from build123d import *

# Parameters (mm, degrees)
SKETCH_1_R      = 11
SKETCH_1_R_2    = 1.5
SKETCH_1_R_3    = 3
EXTRUDE_1_DEPTH = 4


with BuildPart() as part:
    # 草图1 → 凸台-拉伸1 (new body)
    with BuildSketch(Plane.XY):
        with BuildLine():
            Line((-15.909902577, 23.909902577), (15.909902577, 23.909902577))
            ThreePointArc((15.909902577, 23.909902577), (21.566756826, 21.566756826), (23.909902577, 15.909902577))
            Line((23.909902577, 15.909902577), (23.909902577, -15.909902577))
            ThreePointArc((23.909902577, -15.909902577), (21.566756826, -21.566756826), (15.909902577, -23.909902577))
            Line((15.909902577, -23.909902577), (-15.909902577, -23.909902577))
            ThreePointArc((-15.909902577, -23.909902577), (-21.566756826, -21.566756826), (-23.909902577, -15.909902577))
            Line((-23.909902577, -15.909902577), (-23.909902577, 15.909902577))
            ThreePointArc((-23.909902577, 15.909902577), (-21.566756826, 21.566756826), (-15.909902577, 23.909902577))
        make_face()
        Circle(SKETCH_1_R, mode=Mode.SUBTRACT)
        with Locations((0, 14)):
            Circle(SKETCH_1_R_2, mode=Mode.SUBTRACT)
        with Locations((14, 0)):
            Circle(SKETCH_1_R_2, mode=Mode.SUBTRACT)
        with Locations((0, -14)):
            Circle(SKETCH_1_R_2, mode=Mode.SUBTRACT)
        with Locations((-14, 0)):
            Circle(SKETCH_1_R_2, mode=Mode.SUBTRACT)
        with Locations((15.909902577, 15.909902577)):
            Circle(SKETCH_1_R_3, mode=Mode.SUBTRACT)
        with Locations((15.909902577, -15.909902577)):
            Circle(SKETCH_1_R_3, mode=Mode.SUBTRACT)
        with Locations((-15.909902577, -15.909902577)):
            Circle(SKETCH_1_R_3, mode=Mode.SUBTRACT)
        with Locations((-15.909902577, 15.909902577)):
            Circle(SKETCH_1_R_3, mode=Mode.SUBTRACT)
    extrude(amount=EXTRUDE_1_DEPTH)


solid = part.part
The listing builds one solid part. Answer for the finished solid, in the listing's coordinates (mm). Coordinates: 2 decimals unless noted, no trailing zeros. Write each loop counter-clockwise with the first axis right and the second up, starting at its lowest first coordinate (ties: lowest second). Pieces come first, ordered by that corner, then holes. Notation, with made-up numbers: (19.25, 42.25) -> (47.25, 42.25) arc R17 ccw to (47.25, 62.25) -> close; hole circle Ø5 at (32.5, -17). An arc over 180 degrees is marked (long way). One line per question, with ' | ' between items.
1. Section D-D (y = 7.5) is taken. Determine the outline of the cut face in (x, z), and give its area (3 significant figures).
Verdict:
outline: (-23.91, 0) -> (-8.05, 0) -> (-8.05, 4) -> (-23.91, 4) -> close; (8.05, 0) -> (23.91, 0) -> (23.91, 4) -> (8.05, 4) -> close | area: 127 mm^2
2. Section B-B (z = 2.3) is taken. State how many separate pieces and enclosed holes the cut face has, and give its area (3 significant figures).
Verdict:
separate pieces: 1 | enclosed holes: 9 | area: 1,710 mm^2
3. Given pin 1 Ø2 at (y, z) = (18.5, 1.5) entering from -X; pin 2 Ø1 at (x, z) = (-18, 2.5) entering from +Y, each flat-ended and moving along its own axis, determine where each tip first touches the part or whether it passes through.
Verdict:
pin 1: stops at x = -23.75 | pin 2: stops at y = 23.75
4. Straight lines are drawn through the part: line 1 (X direction, y = -16, z = 1.15); line 2 (Y direction, x = 0, z = 3); line 3 (Y direction, x = -14, z = 2.2). For each, find the intervals that lie inside material, in ascending order.
Verdict:
line 1: x = -23.91 to -18.91, -12.91 to 12.91, 18.91 to 23.91 | line 2: y = -23.91 to -15.5, -12.5 to -11, 11 to 12.5, 15.5 to 23.91 | line 3: y = -23.91 to -18.22, -13.6 to -1.5, 1.5 to 13.6, 18.22 to 23.91
5. For a pull along Y with two mould halves and no side action, classify faces 1 (the flat face through (0, 23.91, 2)), 2 (the cylindrical face through (-0.325, 12.536, 1.972)), 3 (the cylindrical face through (21.63, -21.5, 1.97)), 4 (the cylindrical face through (15.26, -18.84, 1.97)) as released by +Y, released by -Y, zero draft, split by the parting line, or undercut.
Verdict:
face 1: released by +Y | face 2: undercut | face 3: released by -Y | face 4: undercut
6. Section A-A (y = 0) is taken. Determine the outline of the cut face in (x, z), and give its area (3 significant figures).
Verdict:
outline: (-23.91, 0) -> (-15.5, 0) -> (-15.5, 4) -> (-23.91, 4) -> close; (-12.5, 0) -> (-11, 0) -> (-11, 4) -> (-12.5, 4) -> close; (11, 0) -> (12.5, 0) -> (12.5, 4) -> (11, 4) -> close; (15.5, 0) -> (23.91, 0) -> (23.91, 4) -> (15.5, 4) -> close | area: 79.3 mm^2
